For this review, use the dimensioned drawing (mm, ordinates from the lowest corner) and the shaded views. Round coordinates to 2 decimals unless told otherwise and drop trailing zeros. Loops run counter-clockwise (first coordinate to the right, second up) from the corner with the lowest first, then second, coordinate; pieces in that order, holes last. Notation, with made-up numbers: M 26.5,-37.75 L 71.5,-37.75 A9 ccw 71.5,-30.75 Z; hole C -8.5,61 d5. An arc over 180 degrees is marked long. Use a Markdown table: item, result. Add a question column.
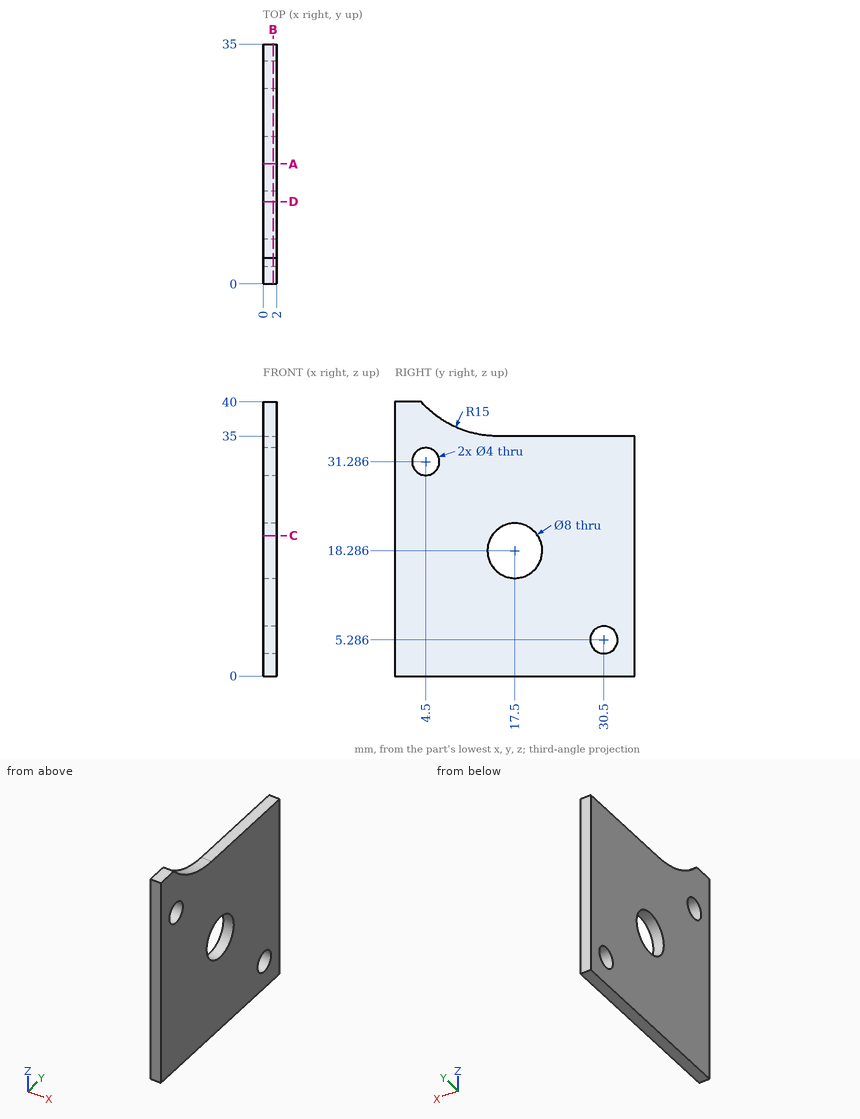
(1) Insertion check: pin 1 Ø1 at (x, y) = (1, 26) entering from +Z; pin 2 Ø7 at (y, z) = (17.5, 18.29) entering from -X. Each pin has a flat end and moves straight along its axis. Give the tip position at first contact, or say it passes through.
(2) Consider section B-B, the plane x = 1.45. Give the boundary of the cut face in (y, z) (1 decimal), then the cut area to 3 significant figures.
(3) To check wall thickness, follow probe 1 along Z at (x, y) = (1.5, 29) (1 decimal); probe 2 along Y at (x, z) = (1.4, 19.5); probe 3 along Y at (x, z) = (1.15, 3.5) (1 decimal). State the ranges of each line that lie inside material, in increasing order.
(4) Consider section A-A, the plane y = 17.5. Give the boundary of the cut face in (x, z) (1 decimal).
(5) Consider section D-D, the plane y = 12. Give the boundary of the cut face in (x, z).
(6) Consider section C-C, the plane z = 20.5. Give the boundary of the cut face in (x, y).
Found:
| question | item | result |
|---|---|---|
| 1 | pin 1 | stops at z = 35 |
| 1 | pin 2 | passes through |
| 2 | outline | M 0,0 L 35,0 L 35,35 L 15,35 A15 cw 3.8,40 L 0,40 Z; hole C 4.5,31.3 d4; hole C 17.5,18.3 d8; hole C 30.5,5.3 d4 |
| 2 | area | 1,190 mm^2 |
| 3 | probe 1 | z = 0 to 4, 6.6 to 35 |
| 3 | probe 2 | y = 0 to 13.69, 21.31 to 35 |
| 3 | probe 3 | y = 0 to 29.6, 31.4 to 35 |
| 4 | outline | M 0,0 L 2,0 L 2,14.3 L 0,14.3 Z; M 0,22.3 L 2,22.3 L 2,35 L 0,35 Z |
| 5 | outline | M 0,0 L 2,0 L 2,35.3 L 0,35.3 Z |
| 6 | outline | M 0,0 L 2,0 L 2,14.17 L 0,14.17 Z; M 0,20.83 L 2,20.83 L 2,35 L 0,35 Z |
